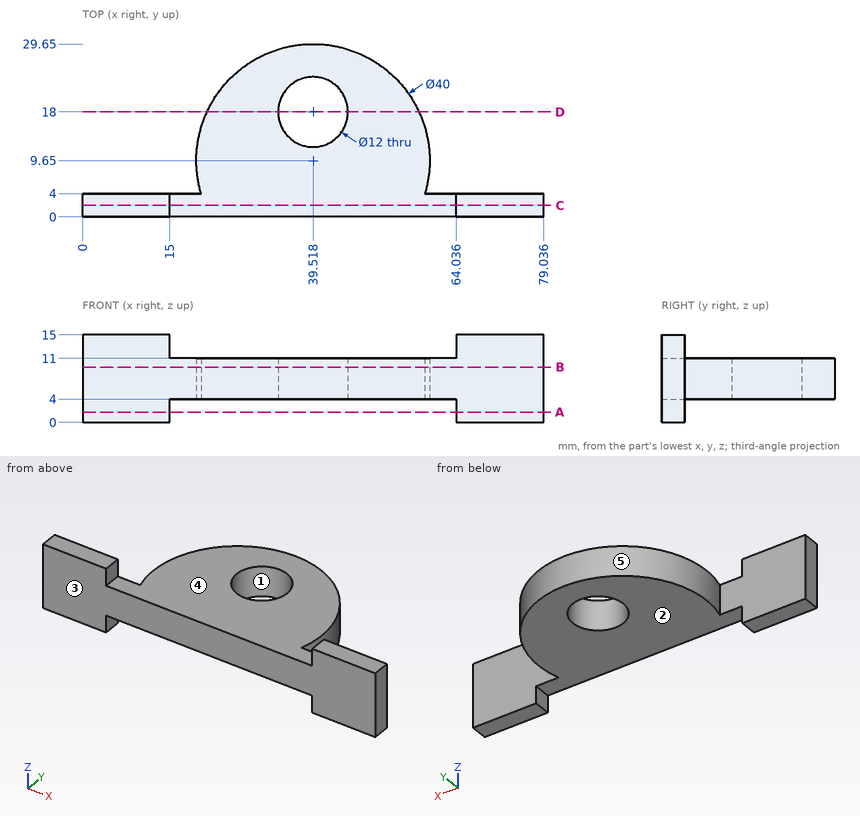
Source: three-view drawing plus pictorial views. Frame: mm from the lowest corner of the part. A direction names the side the tool comes from. Round coordinates to 2 decimals unless told otherwise and drop trailing zeros. Order: outer loops, then holes, each group sorted by start corner. A loop starts at its lowest first (then second) coordinate and runs counter-clockwise, first axis right, second up. Notation, with made-up numbers: (49, -11.5) - (71, -11.5) arc R21 ccw to (71, 5.5) - close; hole circle Ø7 at (9, 54.5). An arc over 180 degrees is marked (long way). Answer in a Markdown table with one row per item.
Item 1: Section query B-B (z = 9.5). Return the cut outline in (x, y), then the cut area to 3 significant figures.
Model answer:
| item | result |
|---|---|
| outline | (0, 0) - (79.04, 0) - (79.04, 4) - (58.7, 4) arc R20 ccw (long way) to (20.33, 4) - (0, 4) - close; hole circle Ø12 at (39.52, 18) |
| area | 1,050 mm² |
Item 2: Line query: line 1 (X direction, y = 3, z = 1.5); line 2 (Y direction, x = 18.5, z = 4.25); line 3 (Z direction, x = 37, y = 7.5). Output: solid intervals per line, ascending.
Model answer:
| item | result |
|---|---|
| line 1 | x = 0 to 15, 64.04 to 79.04 |
| line 2 | y = 0 to 4 |
| line 3 | z = 4 to 11 |
Item 3: Section query C-C (y = 2). Return the cut outline in (x, z).
Model answer:
| item | result |
|---|---|
| outline | (0, 0) - (15, 0) - (15, 4) - (64.04, 4) - (64.04, 0) - (79.04, 0) - (79.04, 15) - (64.04, 15) - (64.04, 11) - (15, 11) - (15, 15) - (0, 15) - close |
Item 4: Pin query (flat end, axial travel): pin 1 (6 mm diameter, centred on y = 21.5, z = 5, fed in from +X); pin 2 (5 mm diameter, centred on x = 23.5, y = 10, fed in from +Z); pin 3 (8 mm diameter, centred on y = 8.5, z = 7, fed in from +X). Return the tip coordinate at first contact, or that it passes through.
Model answer:
| item | result |
|---|---|
| pin 1 | stops at x = 57.45 |
| pin 2 | stops at z = 11 |
| pin 3 | stops at x = 59.52 |
Item 5: Reachability of the marked faces 1 and 2 from +Z, -Z, +X, -X, +Y, -Y: full face, straight path, thin tool, end or side. Return the list, or none.
Model answer:
| item | result |
|---|---|
| face 1 | +Z, -Z |
| face 2 | -Z, +Y, -Y |
Item 6: Mould query, pull axis Y, two halves, no side actions, for the marked faces 3, 4 and 5. Classes: released by +Y, released by -Y, zero draft, split by the parting line, or undercut.
Model answer:
| item | result |
|---|---|
| face 3 | released by -Y |
| face 4 | zero draft |
| face 5 | undercut |
Item 7: Section query D-D (y = 18). Return the cut outline in (x, z).
Model answer:
| item | result |
|---|---|
| outline | (21.34, 4) - (33.52, 4) - (33.52, 11) - (21.34, 11) - close; (45.52, 4) - (57.69, 4) - (57.69, 11) - (45.52, 11) - close |
Item 8: Section query A-A (z = 1.75). Return the cut outline in (x, y), then the cut area to 3 significant figures.
Model answer:
| item | result |
|---|---|
| outline | (0, 0) - (15, 0) - (15, 4) - (0, 4) - close; (64.04, 0) - (79.04, 0) - (79.04, 4) - (64.04, 4) - close |
| area | 120 mm² |
